Can you work these out from the model? Positions are in its coordinate system, mm. A direction names the side the tool comes from. Give positions to 0.01 mm unless a question says otherwise; leave off trailing zeros. Order: outer loops, then holes, each group sorted by start corner. A loop starts at its lowest first (then second) coordinate and runs counter-clockwise, first axis right, second up.
```python
from build123d import *

# Parameters (mm, degrees)
BASE_FLANGE1_DEPTH           = 1.5
EDGE_FLANGE1_STRIP_W         = 9.048
EDGE_FLANGE1_STRIP_H         = 1.5
EDGE_FLANGE1_STRIP_CUT_DEPTH = 42
EDGE_FLANGE1_DEPTH           = 42
SKETCH9_R                    = 12.5
CUT_EXTRUDE1_DEPTH           = 1.5
SKETCH10_R                   = 2.15
CUT_EXTRUDE2_DEPTH           = 67.221899701
SKETCH11_R                   = 1.65
CUT_EXTRUDE3_DEPTH           = 67.221899701
CHAMFER1_SIZE                = 4
CHAMFER2_SIZE                = 3
SKETCH12_W                   = 3.295995972
SKETCH12_H                   = 14
CUT_EXTRUDE4_DEPTH           = 67.221899701
CHAMFER3_SIZE                = 2
SKETCH13_R                   = 1.25
CUT_EXTRUDE5_DEPTH           = 67.221899701
FILLET1_R                    = 0.5


# Sheet-metal steps are written as plain solids
with BuildPart() as part:
    # Sketch1 → Base-Flange1 (new body)
    with BuildSketch(Plane(origin=(0, 0, 0), x_dir=(1, 0, 0), z_dir=(0, 1, 0))):
        Polygon((-21, 43.5), (-5, 43.5), (-5, 20.5), (5, 20.5), (5, 43.5), (21, 43.5), (21, 0), (-21, 0), align=None)
    extrude(amount=-BASE_FLANGE1_DEPTH)

    # Edge-Flange1 strip (across the edge) → Edge-Flange1 strip cut (cut)
    with BuildSketch(Plane(origin=(-21, 0, 0), x_dir=(0, 0, -1), z_dir=(1, 0, 0))):
        with Locations((-1.5, -0.75)):
            Rectangle(EDGE_FLANGE1_STRIP_W, EDGE_FLANGE1_STRIP_H)
    extrude(amount=EDGE_FLANGE1_STRIP_CUT_DEPTH, mode=Mode.SUBTRACT)

    # Edge-Flange1 section (across the edge) → Edge-Flange1 (add)
    with BuildSketch(Plane(origin=(-21, 0, 0), x_dir=(0, 0, -1), z_dir=(1, 0, 0))):
        with BuildLine():
            Line((0, 1.524), (0, 45.3))
            Line((0, 45.3), (1.5, 45.3))
            Line((1.5, 45.3), (1.5, 1.524))
            ThreePointArc((1.5, 1.524), (1.946369265, 0.446369265), (3.024, 0))
            Line((3.024, 0), (3.024, -1.5))
            ThreePointArc((3.024, -1.5), (0.885709094, -0.614290906), (0, 1.524))
        make_face()
    extrude(amount=EDGE_FLANGE1_DEPTH)

    # Sketch9 → Cut-Extrude1 (cut)
    with BuildSketch(Plane.XY):
        with Locations((0, 24.15)):
            Circle(SKETCH9_R)
    extrude(amount=-CUT_EXTRUDE1_DEPTH, mode=Mode.SUBTRACT)

    # Sketch10 → Cut-Extrude2 (cut, through all)
    with BuildSketch(Plane.XY):
        with Locations((-15.5, 39.65)):
            Circle(SKETCH10_R)
        with Locations((15.5, 39.65)):
            Circle(SKETCH10_R)
        with Locations((15.5, 8.65)):
            Circle(SKETCH10_R)
    extrude(amount=-CUT_EXTRUDE2_DEPTH, mode=Mode.SUBTRACT)

    # Sketch11 → Cut-Extrude3 (cut, through all)
    with BuildSketch(Plane(origin=(0, 0, 0), x_dir=(1, 0, 0), z_dir=(0, 1, 0))):
        with Locations(Location((-13, 40, 0), (0, 0, 270))):
            Circle(SKETCH11_R)
        with Locations(Location((13, 40, 0), (0, 0, 90))):
            Circle(SKETCH11_R)
    extrude(amount=-CUT_EXTRUDE3_DEPTH, mode=Mode.SUBTRACT)

    # Chamfer1
    chamfer1_edges = [part.edges().sort_by_distance(p)[0] for p in [
        (-21, 45.3, -0.75),
        (21, 45.3, -0.75),
    ]]
    chamfer(chamfer1_edges, length=CHAMFER1_SIZE)

    # Chamfer2
    chamfer2_edges = [part.edges().sort_by_distance(p)[0] for p in [
        (-21, -0.75, -43.5),
        (-5, -0.75, -43.5),
        (5, -0.75, -43.5),
        (21, -0.75, -43.5),
    ]]
    chamfer(chamfer2_edges, length=CHAMFER2_SIZE)

    # Sketch12 → Cut-Extrude4 (cut, through all)
    with BuildSketch(Plane.XY):
        with Locations((-19.352002014, 13.819078659)):
            Rectangle(SKETCH12_W, SKETCH12_H)
    extrude(amount=-CUT_EXTRUDE4_DEPTH, mode=Mode.SUBTRACT)

    # Chamfer3
    chamfer3_edges = [part.edges().sort_by_distance(p)[0] for p in [
        (-21, 6.819078659, -0.75),
        (-21, 20.819078659, -0.75),
    ]]
    chamfer(chamfer3_edges, length=CHAMFER3_SIZE)

    # Sketch13 → Cut-Extrude5 (cut, through all)
    with BuildSketch(Plane(origin=(0, 0, 0), x_dir=(1, 0, 0), z_dir=(0, 1, 0))):
        with Locations(Location((0, 17.25, 0), (0, 0, 270))):
            Circle(SKETCH13_R)
    extrude(amount=-CUT_EXTRUDE5_DEPTH, mode=Mode.SUBTRACT)

    # Fillet1
    fillet1_edges = [part.edges().sort_by_distance(p)[0] for p in [
        (21, 41.3, -0.75),
        (-8, -0.75, -43.5),
        (-18, -0.75, -43.5),
        (-21, -0.75, -40.5),
        (21, -0.75, -40.5),
        (8, -0.75, -43.5),
        (18, -0.75, -43.5),
        (-5, -0.75, -40.5),
        (5, -0.75, -40.5),
        (-5, -0.75, -20.5),
        (5, -0.75, -20.5),
        (-17.704004028, 20.819078659, -0.75),
        (-17.704004028, 6.819078659, -0.75),
        (-19, 6.819078659, -0.75),
        (-21, 4.819078659, -0.75),
        (-21, 22.819078659, -0.75),
        (-19, 20.819078659, -0.75),
        (-21, 41.3, -0.75),
        (17, 45.3, -0.75),
        (-17, 45.3, -0.75),
    ]]
    fillet(fillet1_edges, radius=FILLET1_R)


solid = part.part
```
1) If I drill on line 1 (X direction, y = -0.4, z = -40); line 2 (Z direction, x = 1, y = 42.5), over which ranges is the centre line in solid material (lowest first)?
2) Suppose I cut it at C-C (y = 39.65). Please give me the cut outline in (x, z).
3) Which directions (+Z, -Z, +X, -X, +Y, -Y) give clear straight access to the entire face, cutting with the end or side of a thin tool? Please do faces 1 (the face through (6.5, -0.7, -42)), 2 (the face through (-19.5, -0.7, -42)).
4) I'm going to push flat-ended pins straight in: pin 1 Ø1 at (x, z) = (1.5, -9) entering from +Y; pin 2 Ø5.5 at (x, y) = (-15.5, 39.65) entering from +Z; pin 3 Ø2.5 at (x, z) = (-13, -40) entering from -Y; pin 4 Ø0.8 at (y, z) = (16, -1) entering from -X. Where does each tip first touch, or does it pass through?
5) Suppose I cut it at B-B (x = 0). Please give me the cut outline in (y, z).
6) Suppose I cut it at D-D (y = 8.65). Please give me the cut outline in (x, z), and give its area (3 significant figures).
7) Suppose I cut it at A-A (z = -17.25). Please give me the cut outline in (x, y).
8) We'd pull the mould along Y, two halves only. Please class faces 3 (the face through (0, 0, -19)), 4 (the face through (16.49, 37.74, -0.74)), 5 (the face through (0, -1.5, -19)), 6 (the face through (14, 23, 0)): +Y half, -Y half, draft (parallel to the pull), parting line (faces both ways), or undercut.
Results:
1. line 1: x = -21 to -14.65, -11.35 to -5, 5 to 11.35, 14.65 to 21
1. line 2: z = -1.5 to 0
2. outline: (-21, -1.5) - (-17.65, -1.5) - (-17.65, 0) - (-21, 0) - close; (-13.35, -1.5) - (13.35, -1.5) - (13.35, 0) - (-13.35, 0) - close; (17.65, -1.5) - (21, -1.5) - (21, 0) - (17.65, 0) - close
3. face 1: -Z, +Y, -Y
3. face 2: -Z, -X, +Y, -Y
4. pin 1: stops at y = 0
4. pin 2: stops at z = 0
4. pin 3: passes through
4. pin 4: stops at x = -17.7
5. outline: (-1.5, -20.5) - (0, -20.5) - (0, -18.5) - (-1.5, -18.5) - close; (-1.5, -16) - (0, -16) - (0, -3.02) arc R1.52 cw to (1.52, -1.5) - (11.65, -1.5) - (11.65, 0) - (1.52, 0) arc R3.02 ccw to (-1.5, -3.02) - close; (36.65, -1.5) - (45.3, -1.5) - (45.3, 0) - (36.65, 0) - close
6. outline: (-17.7, -1.5) - (13.35, -1.5) - (13.35, 0) - (-17.7, 0) - close; (17.65, -1.5) - (21, -1.5) - (21, 0) - (17.65, 0) - close
6. area: 51.6 mm2
7. outline: (-21, -1.5) - (-1.25, -1.5) - (-1.25, 0) - (-21, 0) - close; (1.25, -1.5) - (21, -1.5) - (21, 0) - (1.25, 0) - close
8. face 3: +Y half
8. face 4: undercut
8. face 5: -Y half
8. face 6: draft
